The listing builds one solid part. Answer for the finished solid, in the listing's coordinates (mm). A direction names the side the tool comes from. Coordinates: 2 decimals unless noted, no trailing zeros. Order: outer loops, then holes, each group sorted by start corner. A loop starts at its lowest first (then second) coordinate and runs counter-clockwise, first axis right, second up. Notation, with made-up numbers: (0.25, 39.25) -> (52.25, 39.25) arc R21 ccw to (52.25, 64.25) -> close; hole circle Ø11 at (34.5, -26.75). An arc over 180 degrees is marked (long way). Write each question's results on one line, items separated by ' | '. Start each with the question number.
(1) Straight lines are drawn through the part: L1, parallel to X at y = 0.25, z = -0.35; L2, parallel to Y at x = 4, z = 0.5; L3, parallel to X at y = 4.25, z = -0.45. For each, find the intervals that lie inside material, in ascending order.
(2) The part is cut by section C-C, the plane z = 0.3. Give the vertices of the cut face in (x, y).
(3) The part is cut by section B-B, the plane x = -6. Give the vertices of the cut face in (y, z), then the cut area to 3 significant figures.
(4) A tool of negligible diameter and unlimited length cuts with its end or side. For faces 4 (the face through (-3.413, -5.802, 0.011)), 5 (the face through (-2, -7, 0.794)), from which of +Z, -Z, +X, -X, +Y, -Y can it reach the whole face along a straight path? Write none if from no direction.
(5) The part is cut by section A-A, the plane y = 0. Give the vertices of the cut face in (x, z), then the cut area to 3 significant figures.
(6) Determine the mould class of faces 1 (the face through (-2, -7, -0.794)), 2 (the face through (-1.323, 10.074, 0.011)), 3 (the face through (3.318, -5.856, 0.011)) for opening direction Y: +Y half, -Y half, draft (parallel to the pull), parting line (faces both ways), or undercut.
(7) Given pin 1 (0.5 mm diameter, centred on y = -1.5, z = 0.5, fed in from +X), flat-ended and moving along its own axis, determine where the tip first touches the part or whether it passes through.
```python
from build123d import *

# Parameters (mm, degrees)
SKETCH1_R           = 10.16
BOSS_EXTRUDE1_DEPTH = 0.79375


with BuildPart() as part:
    # Sketch1 → Boss-Extrude1 (new, symmetric)
    with BuildSketch(Plane.XY):
        Circle(SKETCH1_R)
        Polygon((0, 7.772289324), (-6.731, 3.886144662), (-6.731, -3.886144662), (0, -7.772289324), (6.731, -3.886144662), (6.731, 3.886144662), align=None, mode=Mode.SUBTRACT)
    extrude(amount=BOSS_EXTRUDE1_DEPTH, both=True)


solid = part.part
```
Established:
1) L1: x = -10.16 to -6.73, 6.73 to 10.16 | L2: y = -9.34 to -5.46, 5.46 to 9.34 | L3: x = -9.23 to -6.1, 6.1 to 9.23
2) outline: circle Ø20.32 at (0, 0); hole (-6.73, -3.89) -> (0, -7.77) -> (6.73, -3.89) -> (6.73, 3.89) -> (0, 7.77) -> (-6.73, 3.89) -> close
3) outline: (-8.2, -0.79) -> (-4.31, -0.79) -> (-4.31, 0.79) -> (-8.2, 0.79) -> close; (4.31, -0.79) -> (8.2, -0.79) -> (8.2, 0.79) -> (4.31, 0.79) -> close | area: 12.4 mm^2
4) face 4: +Z, -Z | face 5: +Z, +X, -X, +Y, -Y
5) outline: (-10.16, -0.79) -> (-6.73, -0.79) -> (-6.73, 0.79) -> (-10.16, 0.79) -> close; (6.73, -0.79) -> (10.16, -0.79) -> (10.16, 0.79) -> (6.73, 0.79) -> close | area: 10.9 mm^2
6) face 1: draft | face 2: parting line | face 3: undercut
7) pin 1: stops at x = 10.08
